from build123d import *

# Parameters (mm, degrees)
PAD001_DEPTH    = 2.8
POCKET005_DEPTH = 2.801
SKETCH021_W     = 12.7
SKETCH021_H     = 1.6
POCKET010_DEPTH = 2.801


with BuildPart() as part:
    # Sketch001 (on Face18 of ShapeBinder) → Pad001 (new body)
    with BuildSketch(Plane.YZ.offset(35)):
        Polygon((-22.588718, 60.327675), (17.411282, 60.327675), (17.411282, -34.672325), (-57.588718, -34.672325), (-57.588718, 0.327675), (-23.239438, 0.327675), (-7.588718, 43.327675), (-22.588718, 43.327675), align=None)
        with BuildLine():
            ThreePointArc((-12.161797, -2.94822), (-14.851323, 2.819487), (-20.61903, 0.129961))
            Line((-20.61903, 0.129961), (-23.697212, -8.327272))
            ThreePointArc((-23.697212, -8.327272), (-21.007685, -14.09498), (-15.239978, -11.405454))
            Line((-15.239978, -11.405454), (-12.161797, -2.94822))
        make_face(mode=Mode.SUBTRACT)
        with BuildLine():
            ThreePointArc((-3.468033, -5.876244), (-5.261051, -2.031105), (-9.106189, -3.824123))
            Line((-9.106189, -3.824123), (-12.18437, -12.281356))
            ThreePointArc((-12.18437, -12.281356), (-10.391353, -16.126495), (-6.546214, -14.333477))
            Line((-6.546214, -14.333477), (-3.468033, -5.876244))
        make_face(mode=Mode.SUBTRACT)
        Polygon((10.819102, 21.538585), (13.450241, 20.580929), (7.057884, 3.018073), (4.426745, 3.97573), align=None, mode=Mode.SUBTRACT)
        Polygon((1.006544, -5.421196), (3.637683, -6.378853), (-2.754673, -23.941708), (-5.385813, -22.984051), align=None, mode=Mode.SUBTRACT)
    extrude(amount=PAD001_DEPTH)

    # Sketch013 (on Face26 of Pad001) → Pocket005 (cut, through all)
    with BuildSketch(Plane.YZ.offset(37.8)):
        with BuildLine():
            ThreePointArc((1.252746, -5.377784), (0.900889, -5.194619), (0.815033, -5.581893))
            ThreePointArc((0.858445, -5.828095), (0.869723, -5.699178), (0.815033, -5.581893))
            Line((0.858445, -5.828095), (1.413442, -5.569295))
            ThreePointArc((1.252746, -5.377784), (1.307436, -5.495069), (1.413442, -5.569295))
        make_face()
        with BuildLine():
            ThreePointArc((3.681095, -6.625055), (3.86426, -6.273198), (3.476986, -6.187342))
            ThreePointArc((3.230784, -6.230754), (3.359701, -6.242032), (3.476986, -6.187342))
            Line((3.489584, -6.785752), (3.230784, -6.230754))
            ThreePointArc((3.681095, -6.625055), (3.56381, -6.679746), (3.489584, -6.785752))
        make_face()
        with BuildLine():
            ThreePointArc((-5.429225, -22.737849), (-5.61239, -23.089706), (-5.225116, -23.175563))
            ThreePointArc((-4.978914, -23.13215), (-5.107831, -23.120872), (-5.225116, -23.175563))
            Line((-5.237714, -22.577153), (-4.978914, -23.13215))
            ThreePointArc((-5.429225, -22.737849), (-5.31194, -22.683159), (-5.237714, -22.577153))
        make_face()
        with BuildLine():
            ThreePointArc((-3.000875, -23.98512), (-2.649019, -24.168285), (-2.563162, -23.781011))
            ThreePointArc((-2.606574, -23.534809), (-2.617853, -23.663726), (-2.563162, -23.781011))
            Line((-2.606574, -23.534809), (-3.161572, -23.793609))
            ThreePointArc((-3.000875, -23.98512), (-3.055566, -23.867835), (-3.161572, -23.793609))
        make_face()
        with BuildLine():
            ThreePointArc((11.065304, 21.581997), (10.713447, 21.765162), (10.62759, 21.377888))
            ThreePointArc((10.671003, 21.131686), (10.682281, 21.260603), (10.62759, 21.377888))
            Line((10.671003, 21.131686), (11.226, 21.390486))
            ThreePointArc((11.065304, 21.581997), (11.119994, 21.464712), (11.226, 21.390486))
        make_face()
        with BuildLine():
            ThreePointArc((13.493653, 20.334727), (13.676818, 20.686583), (13.289544, 20.77244))
            ThreePointArc((13.043342, 20.729028), (13.172259, 20.717749), (13.289544, 20.77244))
            Line((13.302142, 20.17403), (13.043342, 20.729028))
            ThreePointArc((13.493653, 20.334727), (13.376368, 20.280036), (13.302142, 20.17403))
        make_face()
        with BuildLine():
            ThreePointArc((4.383333, 4.221932), (4.200168, 3.870075), (4.587442, 3.784219))
            ThreePointArc((4.833644, 3.827631), (4.704727, 3.83891), (4.587442, 3.784219))
            Line((4.574844, 4.382629), (4.833644, 3.827631))
            ThreePointArc((4.383333, 4.221932), (4.500618, 4.276623), (4.574844, 4.382629))
        make_face()
        with BuildLine():
            ThreePointArc((6.811682, 2.974661), (7.163539, 2.791497), (7.249396, 3.17877))
            ThreePointArc((7.205983, 3.424972), (7.194705, 3.296055), (7.249396, 3.17877))
            Line((7.205983, 3.424972), (6.650986, 3.166173))
            ThreePointArc((6.811682, 2.974661), (6.756992, 3.091946), (6.650986, 3.166173))
        make_face()
    extrude(amount=-POCKET005_DEPTH, mode=Mode.SUBTRACT)

    # Sketch021 (on Face5 of Pocket005) → Pocket010 (cut, through all)
    with BuildSketch(Plane.YZ.offset(37.8)):
        with Locations((-41.903927, -5.472325)):
            Rectangle(SKETCH021_W, SKETCH021_H)
    extrude(amount=-POCKET010_DEPTH, mode=Mode.SUBTRACT)


solid = part.part
The model under review builds one solid part; all positions refer to its coordinate system, in mm. A direction names the side the tool comes from. Give positions to 0.01 mm unless a question says otherwise; leave off trailing zeros. Order: outer loops, then holes, each group sorted by start corner. A loop starts at its lowest first (then second) coordinate and runs counter-clockwise, first axis right, second up. Notation, with made-up numbers: M 40.25,-38 L 75.25,-38 A17 cw 75.25,-33 Z; hole C -2.75,-25 d9. An arc over 180 degrees is marked long. One line per question, with ' | ' between items. Start each with the question number.
1) Consider section C-C, the plane y = -17. Give the boundary of the cut face in (x, z), then the cut area to 3 significant figures.
2) Consider section D-D, the plane z = 46. Give the boundary of the cut face in (x, y).
3) Consider section B-B, the plane x = 37.1. State how many separate pieces and enclosed holes the cut face has, then the cut area to 3 significant figures.
4) Mouldability with a two-part tool opening along Z and no side actions: class faces 3 (the face through (36, -57.589, -17)), 4 (the face through (36, -3, 60.328)), 5 (the face through (36.38, 5.76, 3.49)) as pulls with the +Z half, pulls with the -Z half, needs draft (parallel to the pull), parting line crosses it, or undercut.
5) Wall thickness on L1, parallel to Z at x = 35.25, y = -42.5; L2, parallel to Y at x = 36.7, z = -11.5; L3, parallel to Y at x = 35.8, z = -4: over which ranges is each line inside the solid? List them lowest first. Write a range as from..to.
6) Consider section A-A, the plane z = 12.5. Give the boundary of the cut face in (x, y).
7) For faces 1 (the face through (36.38, -15.524, 21.527)), 2 (the face through (36.38, 7.58, 12.64)), list the 3-axis set-ups (+Z, -Z, +X, -X, +Y, -Y) from which the entire face can be reached by the end or side of a thin tool; tool diameter is ignored.
8) Clearance check with a flat-ended pin moving along its axis: P1, Ø0.8, axis at x = 35.5, y = -47, coming from the +Z side. State where the tip first meets the part, or that it passes through.
Found:
1) outline: M 35,-34.67 L 37.8,-34.67 L 37.8,-13.63 L 35,-13.63 Z; M 35,3.05 L 37.8,3.05 L 37.8,17.47 L 35,17.47 Z; M 35,43.33 L 37.8,43.33 L 37.8,60.33 L 35,60.33 Z | area: 147 mm²
2) outline: M 35,-22.59 L 37.8,-22.59 L 37.8,17.41 L 35,17.41 Z
3) separate pieces: 1 | enclosed holes: 5 | area: 4,360 mm²
4) face 3: needs draft | face 4: pulls with the +Z half | face 5: undercut
5) L1: z = -34.67..-6.27, -4.67..0.33 | L2: y = -57.59..-23.66, -15.28..-11.9, -5.51..-1.21, 1.77..17.41 | L3: y = -57.59..-22.12, -12.54..-9.17, -3.41..17.41
6) outline: M 35,-18.81 L 37.8,-18.81 L 37.8,7.53 L 35,7.53 Z; M 35,10.51 L 37.8,10.51 L 37.8,17.41 L 35,17.41 Z
7) face 1: +X, -X, -Y | face 2: +X, -X
8) P1: stops at z = 0.33
